Could you check a few things on this model? Use its own coordinates, in mm. Face numbers are marked on the shaded views. Give positions to 0.01 mm unless a question says otherwise; leave off trailing zeros. Loops run counter-clockwise (first coordinate to the right, second up) from the corner with the lowest first, then second, coordinate; pieces in that order, holes last. Notation, with made-up numbers: (77.5, 42.5) - (94.5, 42.5) arc R25 ccw to (94.5, 70.5) - close; hole circle Ø5 at (45, -2). An arc over 180 degrees is marked (long way). Answer in a Markdown table with one row per item. Add a question column.
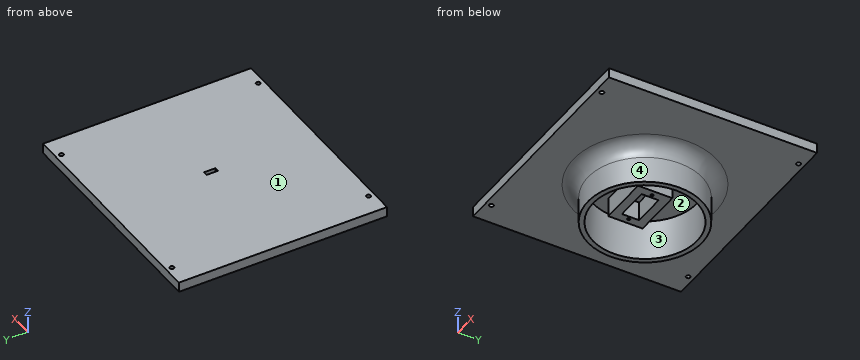
```python
from build123d import *

# Parameters (mm, degrees)
SCHIZZO1_W                   = 160
SCHIZZO1_H                   = 146
SCHIZZO1_R                   = 1.5
ESTRUSIONE_ESTRUSIONE1_DEPTH = 7
SCHIZZO2_W                   = 35
SCHIZZO2_H                   = 24
SCHIZZO2_W_2                 = 23
SCHIZZO2_H_2                 = 12
ESTRUSIONE_ESTRUSIONE2_DEPTH = 13.5
SCHIZZO3_R                   = 1
TAGLIO_ESTRUSIONE1_DEPTH     = 5
SCHIZZO4_R                   = 40
SCHIZZO4_R_2                 = 36.5
ESTRUSIONE_ESTRUSIONE3_DEPTH = 28.5
RACCORDO1_R                  = 10
SCHIZZO5_W                   = 3
SCHIZZO5_H                   = 8
TAGLIO_ESTRUSIONE2_DEPTH     = 41


with BuildPart() as part:
    # Schizzo1 → Estrusione-Estrusione1 (new body)
    with BuildSketch(Plane.XY):
        with Locations((-3.483874863, 6.01)):
            Rectangle(SCHIZZO1_W, SCHIZZO1_H)
        with Locations((-68.483874863, 75.01)):
            Circle(SCHIZZO1_R, mode=Mode.SUBTRACT)
        with Locations((61.516125137, 75.01)):
            Circle(SCHIZZO1_R, mode=Mode.SUBTRACT)
        with Locations((-68.483874863, -62.99)):
            Circle(SCHIZZO1_R, mode=Mode.SUBTRACT)
        with Locations((61.516125137, -62.99)):
            Circle(SCHIZZO1_R, mode=Mode.SUBTRACT)
    extrude(amount=ESTRUSIONE_ESTRUSIONE1_DEPTH)

    # Schizzo2 → Estrusione-Estrusione2 (add)
    with BuildSketch(Plane(origin=(0, 0, 0), x_dir=(-1, 0, 0), z_dir=(0, 0, -1))):
        with Locations((8.983874863, 6.01)):
            Rectangle(SCHIZZO2_W, SCHIZZO2_H)
        with Locations((8.983874863, 6.01)):
            Rectangle(SCHIZZO2_W_2, SCHIZZO2_H_2, mode=Mode.SUBTRACT)
    extrude(amount=ESTRUSIONE_ESTRUSIONE2_DEPTH)

    # Schizzo3 → Taglio-Estrusione1 (cut)
    with BuildSketch(Plane(origin=(0, 0, -13.5), x_dir=(-1, 0, 0), z_dir=(0, 0, -1))):
        with Locations((22.733874863, 6.01)):
            Circle(SCHIZZO3_R)
        with Locations(Location((-4.766125137, 6.01, 0), (0, 0, 180))):
            Circle(SCHIZZO3_R)
    extrude(amount=-TAGLIO_ESTRUSIONE1_DEPTH, mode=Mode.SUBTRACT)

    # Schizzo4 → Estrusione-Estrusione3 (add)
    with BuildSketch(Plane(origin=(0, 0, 0), x_dir=(-1, 0, 0), z_dir=(0, 0, -1))):
        with Locations(Location((3.483874863, 6.01, 0), (0, 0, 180))):
            Circle(SCHIZZO4_R)
        with Locations(Location((3.483874863, 6.01, 0), (0, 0, 180))):
            Circle(SCHIZZO4_R_2, mode=Mode.SUBTRACT)
    extrude(amount=ESTRUSIONE_ESTRUSIONE3_DEPTH)

    # Raccordo1
    raccordo1_edges = [part.edges().sort_by_distance(p)[0] for p in [
        (-43.483874863, 6.01, 0),
    ]]
    fillet(raccordo1_edges, radius=RACCORDO1_R)

    # Schizzo5 → Taglio-Estrusione2 (cut)
    with BuildSketch(Plane(origin=(0, 0, 0), x_dir=(-1, 0, 0), z_dir=(0, 0, -1))):
        with Locations((-1.016125137, 6.01)):
            Rectangle(SCHIZZO5_W, SCHIZZO5_H)
    extrude(amount=-TAGLIO_ESTRUSIONE2_DEPTH, mode=Mode.SUBTRACT)


solid = part.part
```
(1) Please list where these lines run through material, in increasing order: line 1 (X direction, y = 75.01, z = 2); line 2 (Y direction, x = 62.5, z = 4.5); line 3 (X direction, y = -62, z = 5).
(2) We'd pull the mould along Y, two halves only. Please class the marked faces 1, 2, 3 and 4: pulls with the +Y half, pulls with the -Y half, needs draft (parallel to the pull), parting line crosses it, or undercut.
(3) For pin 1 Ø0.6 at (x, y) = (-23, 5.5) entering from -Z; pin 2 Ø4 at (x, z) = (33, -9) entering from +Y; pin 3 Ø12 at (y, z) = (20.5, -20) entering from +X, each with a flat end and sliding along its axis, tell me the tip position at first contact or that it passes through.
(4) I want a section at A-A on z = -25. Please give me the cut outline in (x, y).
Reported:
| question | item | result |
|---|---|---|
| 1 | line 1 | -83.48 to -69.98, -66.98 to 60.02, 63.02 to 76.52 |
| 1 | line 2 | -66.99 to -64.12, -61.86 to 73.88, 76.14 to 79.01 |
| 1 | line 3 | -83.48 to -69.61, -67.36 to 60.39, 62.64 to 76.52 |
| 2 | face 1 | needs draft |
| 2 | face 2 | undercut |
| 2 | face 3 | undercut |
| 2 | face 4 | parting line crosses it |
| 3 | pin 1 | z = -8.5 |
| 3 | pin 2 | y = 26.41 |
| 3 | pin 3 | x = 35.6 |
| 4 | outline | circle Ø80 at (-3.48, 6.01); hole circle Ø73 at (-3.48, 6.01) |
